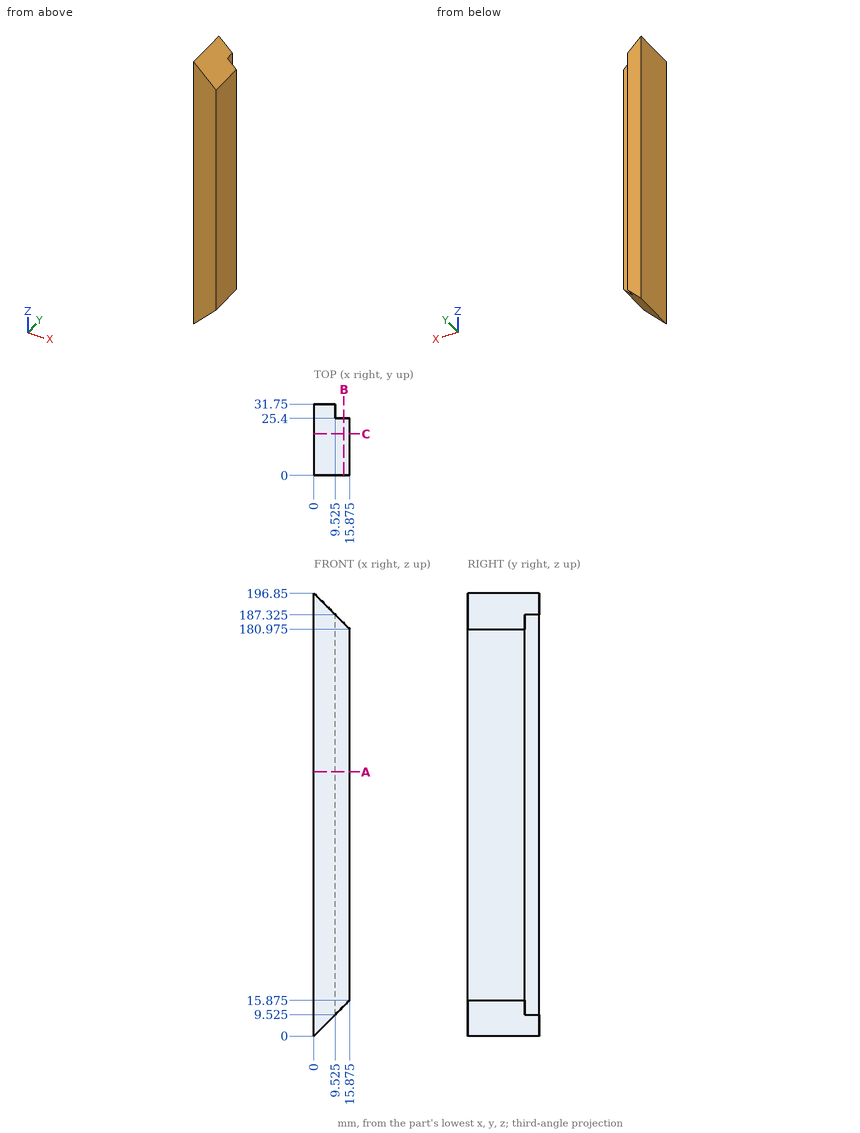
The drawing under review shows one solid part. Ordinate dimensions are in mm from its lowest x, y, z. Give positions to 0.01 mm unless a question says otherwise; leave off trailing zeros. Order: outer loops, then holes, each group sorted by start corner. A loop starts at its lowest first (then second) coordinate and runs counter-clockwise, first axis right, second up. Notation, with made-up numbers: (17, 77.5) -> (36, 77.5) arc R20 ccw to (36, 114.5) -> close; hole circle Ø1 at (-32.75, -22). An arc over 180 degrees is marked (long way). Write item = value, one per line. Start each with the question number.
(1) We need section B-B on x = 13.25. Write out the cut boundary in (y, z).
(2) For pin 1 (1.5 mm diameter, centred on x = 6, y = 22, fed in from +Z); pin 2 (3 mm diameter, centred on x = 11.5, z = 69, fed in from +Y); pin 3 (5 mm diameter, centred on y = 30, z = 58, fed in from +X) (3 decimals), all flat-tipped, find the tip position at first contact; note any pin that passes through.
(3) To check wall thickness, follow line 1 along X through (y, z) = (30, 106) (3 decimals); line 2 along Y through (x, z) = (14, 130.5); line 3 along Z through (x, y) = (4.5, 13). State the ranges of each line that lie inside material, in increasing order.
(4) We need section A-A on z = 117.5. Write out the cut boundary in (x, y) (3 decimals), plus the area to 3 significant figures.
(5) We need section C-C on y = 18.5. Write out the cut boundary in (x, z) (3 decimals), plus the area to 3 significant figures.
Numbers:
q1.outline = (0, 13.25) -> (25.4, 13.25) -> (25.4, 183.6) -> (0, 183.6) -> close
q2.pin_1 = 191.6
q2.pin_2 = 25.4
q2.pin_3 = 9.525
q3.line_1 = 0 to 9.525
q3.line_2 = 0 to 25.4
q3.line_3 = 4.5 to 192.35
q4.outline = (0, 0) -> (15.875, 0) -> (15.875, 25.4) -> (9.525, 25.4) -> (9.525, 31.75) -> (0, 31.75) -> close
q4.area = 464 mm^2
q5.outline = (0, 0) -> (15.875, 15.875) -> (15.875, 180.975) -> (0, 196.85) -> close
q5.area = 2,870 mm^2
